The listing builds one solid part. Answer for the finished solid, in the listing's coordinates (mm). A direction names the side the tool comes from. Give positions to 0.01 mm unless a question says otherwise; leave off trailing zeros. Order: outer loops, then holes, each group sorted by start corner. A loop starts at its lowest first (then second) coordinate and runs counter-clockwise, first axis right, second up. Notation, with made-up numbers: (-6, -16.75) - (23, -16.75) arc R12 ccw to (23, -4.75) - close; hole circle Ø11 at (78, 40.25). An arc over 180 degrees is marked (long way). Answer as a JSON object with one key per item and string values. Group by question number.
Q1. The mould has two halves that part along Z. Classify faces 1 (the face through (-22.1, -5, 6.6)), 2 (the face through (19, 1, 0)), 3 (the face through (45.57, 32.41, 5.23)): released by +Z, released by -Z, zero draft, split by the parting line, or undercut.
Q2. For faces 4 (the face through (15.371, 32.414, 4.944)), 5 (the face through (-25.7, 19, 9)), 6 (the face through (-23, 5, 7)), 7 (the face through (-14, 30.836, 9)), 8 (the face through (58.126, 2.945, 9.86)), determine the directions among +Z, -Z, +X, -X, +Y, -Y from which every point of the face is accessible in a straight line to the end or side of a thin tool.
Q3. A cutting plane is placed at C-C, the plane y = -14. Give the vertices of the cut face in (x, z).
Q4. A cutting plane is placed at D-D, the plane y = 10. Give the vertices of the cut face in (x, z), and give its area (3 significant figures).
Q5. Given pin 1 (12 mm diameter, centred on x = -15, z = 12.5, fed in from -Y); pin 2 (2 mm diameter, centred on x = 16.3, z = 6.4, fed in from +Y); pin 3 (2 mm diameter, centred on x = -12, z = 16, fed in from -Y), each flat-ended and moving along its own axis, determine where each tip first touches the part or whether it passes through.
Q6. Consider line 1 (X direction, y = 17.5, z = 0.25); line 2 (Y direction, x = 32.5, z = 15.75); line 3 (Y direction, x = -10, z = 17). Determine where each line is inside the solid, lowest interval first.
Q7. A cutting plane is placed at B-B, the plane x = -17.7. Give the vertices of the cut face in (y, z), and give its area (3 significant figures).
Q8. A cutting plane is placed at A-A, the plane x = 0. Give the vertices of the cut face in (y, z).
from build123d import *

# Parameters (mm, degrees)
BOSS_EXTRUDE1_DEPTH       = 20
BOSS_EXTRUDE2_START       = 1.6
BOSS_EXTRUDE2_DEPTH       = 1.6
CUT_EXTRUDE1_REACH        = 75.397
CUT_EXTRUDE3_REACH        = 75.397
CUT_EXTRUDE4_REACH        = 75.397
SKETCH6_R                 = 15
F_8_32_TAPPED_HOLE1_D     = 3.4544
F_8_32_TAPPED_HOLE1_DEPTH = 3.2


with BuildPart() as part:
    # Sketch1 → Boss-Extrude1 (new body)
    with BuildSketch(Plane.XY):
        with BuildLine():
            Line((37.281598718, -23.36075752), (1.645598718, -25.647261157))
            ThreePointArc((1.645598718, -25.647261157), (-17.581213168, -18.745424602), (-25.7, 0))
            Line((-25.7, 0), (-25.7, 34.036))
            Line((-25.7, 34.036), (50, 34.036))
            Line((50, 34.036), (59.262043429, 12.400853436))
            ThreePointArc((59.262043429, 12.400853436), (57.530912166, -11.170941189), (37.281598718, -23.36075752))
        make_face()
        with BuildLine():
            ThreePointArc((16.941307547, 14.806826081), (-22.453827861, -1.440699267), (18.694692453, -12.520322444))
            ThreePointArc((18.694692453, -12.520322444), (58.089827861, 3.727202903), (16.941307547, 14.806826081))
        make_face(mode=Mode.SUBTRACT)
    extrude(amount=BOSS_EXTRUDE1_DEPTH)

    # Sketch2 → Boss-Extrude2 (add)
    with BuildSketch(Plane(origin=(0, 0, 0), x_dir=(-1, 0, 0), z_dir=(0, 0, -1)).offset(BOSS_EXTRUDE2_START)):
        with BuildLine():
            Line((25.7, 0), (25.7, 34.036))
            Line((25.7, 34.036), (-50, 34.036))
            Line((-50, 34.036), (-59.262043429, 12.400853436))
            ThreePointArc((-59.262043429, 12.400853436), (-57.530912166, -11.170941189), (-37.281598718, -23.36075752))
            Line((-37.281598718, -23.36075752), (-1.645598718, -25.647261157))
            ThreePointArc((-1.645598718, -25.647261157), (17.581213168, -18.745424602), (25.7, 0))
        make_face()
    extrude(amount=-BOSS_EXTRUDE2_DEPTH)

    # Sketch3 → Cut-Extrude1 (cut, up to next)
    with BuildSketch(Plane.XY.offset(20), mode=Mode.PRIVATE) as cut_extrude1_sk1:
        with BuildLine():
            ThreePointArc((-5.394176999, 25.127531803), (-15.326311164, 20.629934225), (-22.5, 12.419339757))
            Line((-22.5, 12.419339757), (-22.5, 30.836))
            Line((-22.5, 30.836), (-6, 30.836))
            ThreePointArc((-6, 30.836), (-3.129737352, 28.254231355), (-5.394176999, 25.127531803))
        make_face()
    cut_extrude1_tool1 = extrude(cut_extrude1_sk1.sketch, amount=-CUT_EXTRUDE1_REACH, mode=Mode.PRIVATE) & part.part
    # Sketch3 → Cut-Extrude1 (cut, up to next)
    with BuildSketch(Plane.XY.offset(20), mode=Mode.PRIVATE) as cut_extrude1_sk2:
        with BuildLine():
            ThreePointArc((16.634374037, 19.590497707), (11.35689006, 23.054523378), (5.394176999, 25.127531803))
            ThreePointArc((5.394176999, 25.127531803), (3.129737352, 28.254231355), (6, 30.836))
            Line((6, 30.836), (45.922585437, 30.836))
            ThreePointArc((45.922585437, 30.836), (48.2805699, 27.988887856), (45.044015862, 26.202591058))
            ThreePointArc((45.044015862, 26.202591058), (29.810256845, 27.317498757), (16.634374037, 19.590497707))
        make_face()
    cut_extrude1_tool2 = extrude(cut_extrude1_sk2.sketch, amount=-CUT_EXTRUDE1_REACH, mode=Mode.PRIVATE) & part.part
    add(cut_extrude1_tool1.solids().sort_by_distance((-15.04252, 25.299031, 20))[0], mode=Mode.SUBTRACT)
    add(cut_extrude1_tool2.solids().sort_by_distance((22.114051, 27.528579, 20))[0], mode=Mode.SUBTRACT)

    # Sketch5 → Cut-Extrude3 (cut, up to next)
    with BuildSketch(Plane(origin=(0, 0, -1.6), x_dir=(-1, 0, 0), z_dir=(0, 0, -1)), mode=Mode.PRIVATE) as cut_extrude3_sk1:
        with BuildLine():
            Line((25.7, 5), (0, 5))
            ThreePointArc((0, 5), (-5, 0), (0, -5))
            Line((0, -5), (25.20892699, -5))
            ThreePointArc((25.20892699, -5), (25.576937108, -2.512028697), (25.7, 0))
            Line((25.7, 0), (25.7, 5))
        make_face()
    cut_extrude3_tool1 = extrude(cut_extrude3_sk1.sketch, amount=-CUT_EXTRUDE3_REACH, mode=Mode.PRIVATE) & part.part
    add(cut_extrude3_tool1.solids().sort_by_distance((-10.824957, 0.010355, -1.6))[0], mode=Mode.SUBTRACT)

    # Sketch6 → Cut-Extrude4 (cut, up to next)
    with BuildSketch(Plane(origin=(0, 0, -1.6), x_dir=(-1, 0, 0), z_dir=(0, 0, -1)), mode=Mode.PRIVATE) as cut_extrude4_sk1:
        with Locations((-35.636, 2.286503637)):
            Circle(SKETCH6_R)
    cut_extrude4_tool1 = extrude(cut_extrude4_sk1.sketch, amount=-CUT_EXTRUDE4_REACH, mode=Mode.PRIVATE) & part.part
    # Sketch6 → Cut-Extrude4 (cut, up to next)
    with BuildSketch(Plane(origin=(0, 0, -1.6), x_dir=(-1, 0, 0), z_dir=(0, 0, -1)), mode=Mode.PRIVATE) as cut_extrude4_sk2:
        Circle(SKETCH6_R)
    cut_extrude4_tool2 = extrude(cut_extrude4_sk2.sketch, amount=-CUT_EXTRUDE4_REACH, mode=Mode.PRIVATE) & part.part
    add(cut_extrude4_tool1.solids().sort_by_distance((35.636, 2.286504, -1.6))[0], mode=Mode.SUBTRACT)
    add(cut_extrude4_tool2.solids().sort_by_distance((0, 0, -1.6))[0], mode=Mode.SUBTRACT)

    # #8-32 Tapped Hole1
    with Locations(Plane(origin=(0, 34.036, 0), x_dir=(1, 0, 0), z_dir=(0, 1, 0))):
        with Locations((16.3, -6.4), (-17.7, -6.4), (44.3, -6.4)):
            Hole(F_8_32_TAPPED_HOLE1_D / 2, depth=F_8_32_TAPPED_HOLE1_DEPTH)


solid = part.part
Reply:
{
 "1": {"face 1": "zero draft", "face 2": "released by +Z", "face 3": "undercut"},
 "2": {"face 4": "+Y", "face 5": "+Z, -Z, -X, +Y, -Y", "face 6": "+Z, -Z, -X", "face 7": "+Z, -Z", "face 8": "+Z"},
 "3": {"outline": "(-21.55, -1.6) - (-5.39, -1.6) - (-5.39, 0) - (-17.61, 0) - (-17.61, 20) - (-21.55, 20) - close; (5.39, -1.6) - (55.52, -1.6) - (55.52, 20) - (51.16, 20) - (51.16, 0) - (20.11, 0) - (20.11, 20) - (17.61, 20) - (17.61, 0) - (5.39, 0) - close"},
 "4": {"outline": "(-25.7, -1.6) - (-11.18, -1.6) - (-11.18, 0) - (-20.16, 0) - (-20.16, 20) - (-25.7, 20) - close; (11.18, -1.6) - (22.77, -1.6) - (22.77, 0) - (11.18, 0) - close; (48.5, -1.6) - (60.15, -1.6) - (60.15, 20) - (56.77, 20) - (56.77, 0) - (48.5, 0) - close", "area": "239 mm^2"},
 "5": {"pin 1": "stops at y = -24.07", "pin 2": "stops at y = 20.65", "pin 3": "stops at y = -23.23"},
 "6": {"line 1": "x = -25.7 to -22.5, -18.82 to -14.14, 14.14 to 19.06, 52.21 to 57.08", "line 2": "y = -23.67 to -19.99, 24.57 to 27.79, 30.84 to 34.04", "line 3": "y = -23.67 to -20.16, 20.16 to 23.67, 30.84 to 34.04"},
 "7": {"outline": "(-18.63, -1.6) - (-5, -1.6) - (-5, 0) - (-13.89, 0) - (-13.89, 20) - (-18.63, 20) - close; (5, -1.6) - (18.63, -1.6) - (18.63, 20) - (13.89, 20) - (13.89, 0) - (5, 0) - close; (30.84, -1.6) - (34.04, -1.6) - (34.04, 4.67) - (30.84, 4.67) - close; (30.84, 8.13) - (34.04, 8.13) - (34.04, 20) - (30.84, 20) - close", "area": "291 mm^2"},
 "8": {"outline": "(-25.7, -1.6) - (-15, -1.6) - (-15, 0) - (-22.5, 0) - (-22.5, 20) - (-25.7, 20) - close; (15, -1.6) - (34.04, -1.6) - (34.04, 20) - (22.5, 20) - (22.5, 0) - (15, 0) - close"}
}
